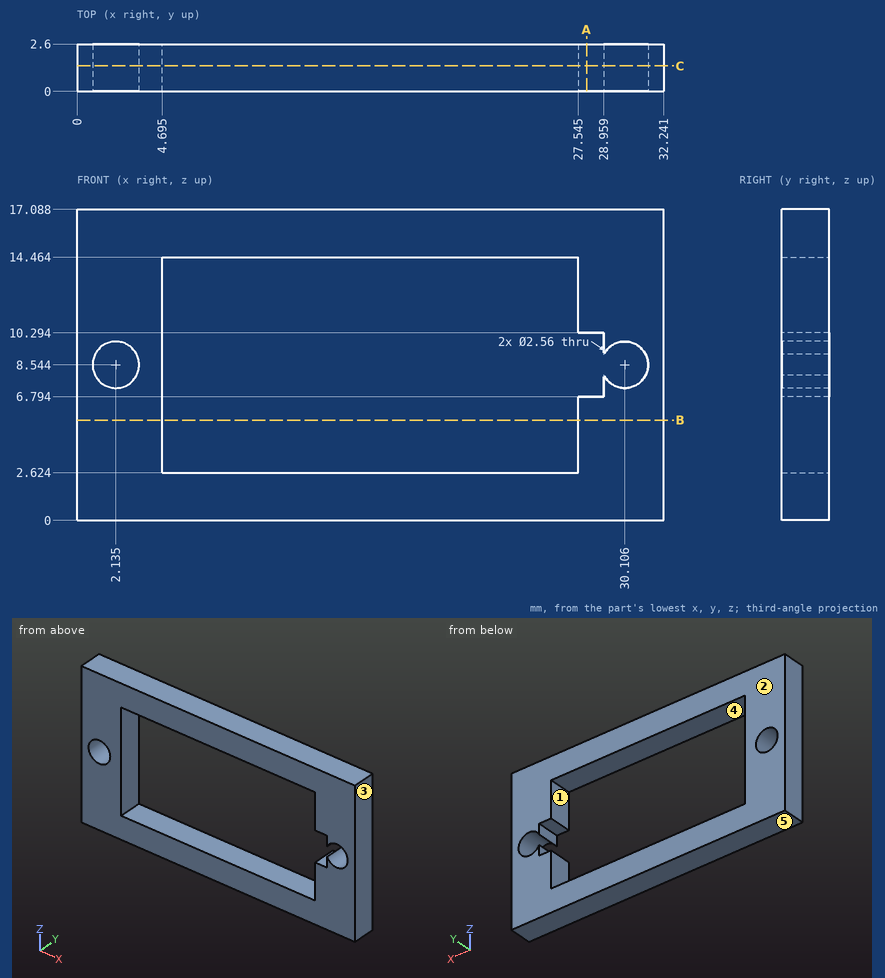
Print and shaded views of the part. All mm, measured from the part's lowest x, y and z. A direction names the side the tool comes from. Coordinates: 2 decimals unless noted, no trailing zeros. Write each loop counter-clockwise with the first axis right and the second up, starting at its lowest first coordinate (ties: lowest second). Pieces come first, ordered by that corner, then holes.
(1) Cut at C-C, the plane y = 1.4. List the corners of the cut face in (x, z) (1 decimal).
(2) Two-plate mould, pull along X, no slides. Class the marked faces 1, 2 and 3: +X half, -X half, draft (parallel to the pull), parting line (faces both ways), or undercut.
(3) Drill centre lines: probe 1 along Z at (x, y) = (12, 1.85); probe 2 along X at (y, z) = (2.45, 7) (1 decimal); probe 3 along X at (y, z) = (0.1, 3.25) (1 decimal). Where is each one in solid material? Low to high.
(4) Cut at B-B, the plane z = 5.5. List the corners of the cut face in (x, y) (1 decimal).
(5) Cut at A-A, the plane x = 28. List the corners of the cut face in (y, z).
(6) 3-axis set-ups, long thin cutter, end or side, ignore diameter. For the marked faces 4 and 5: which of +Z, -Z, +X, -X, +Y, -Y reach the whole face in a straight line?
Geometry says:
1. outline: (0, 0) - (32.2, 0) - (32.2, 17.1) - (0, 17.1) - close; hole circle Ø2.6 at (2.1, 8.5); hole (4.7, 2.6) - (27.5, 2.6) - (27.5, 6.8) - (29, 6.8) - (29, 8) arc R1.3 ccw (long way) to (29, 9.1) - (29, 10.3) - (27.5, 10.3) - (27.5, 14.5) - (4.7, 14.5) - close
2. face 1: undercut
2. face 2: draft
2. face 3: +X half
3. probe 1: z = 0 to 2.62, 14.46 to 17.09
3. probe 2: x = 0 to 4.7, 29 to 32.2
3. probe 3: x = 0 to 4.7, 27.5 to 32.2
4. outline: (0, 0) - (4.7, 0) - (4.7, 2.6) - (0, 2.6) - close; (27.5, 0) - (32.2, 0) - (32.2, 2.6) - (27.5, 2.6) - close
5. outline: (0, 0) - (2.6, 0) - (2.6, 6.79) - (0, 6.79) - close; (0, 10.29) - (2.6, 10.29) - (2.6, 17.09) - (0, 17.09) - close
6. face 4: +Y, -Y
6. face 5: -Z, +X, -X, +Y, -Y
